```python
from build123d import *

# Parameters (mm, degrees)
SKETCH1_R           = 5
SKETCH1_R_2         = 1
SKETCH1_W           = 22
SKETCH1_H           = 12
BOSS_EXTRUDE1_DEPTH = 4


with BuildPart() as part:
    # Sketch1 → Boss-Extrude1 (new body)
    with BuildSketch(Plane.XY):
        with BuildLine():
            Line((0, 15), (200, 12.5))
            ThreePointArc((200, 12.5), (212.5, 0), (200, -12.5))
            Line((200, -12.5), (0, -15))
            ThreePointArc((0, -15), (-15, 0), (0, 15))
        make_face()
        Circle(SKETCH1_R, mode=Mode.SUBTRACT)
        with Locations((208.5, 0)):
            Circle(SKETCH1_R_2, mode=Mode.SUBTRACT)
        with Locations((181.5, 0)):
            Circle(SKETCH1_R_2, mode=Mode.SUBTRACT)
        with Locations((195, 0)):
            Rectangle(SKETCH1_W, SKETCH1_H, mode=Mode.SUBTRACT)
    extrude(amount=BOSS_EXTRUDE1_DEPTH)


solid = part.part
```
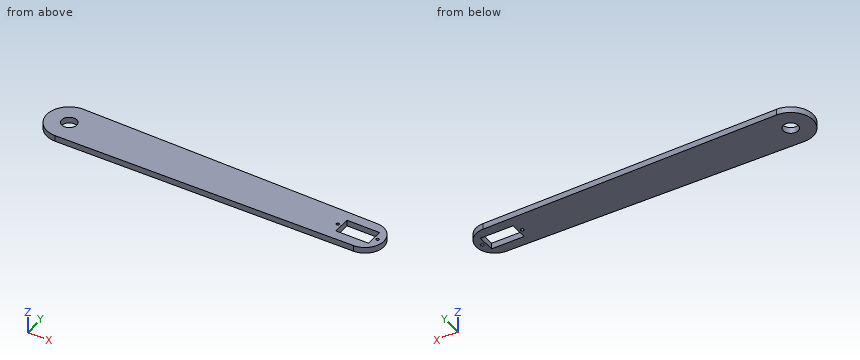
Can you work these out from the model? Positions are in its coordinate system, mm. Round coordinates to 2 decimals unless told otherwise and drop trailing zeros. Order: outer loops, then holes, each group sorted by start corner. A loop starts at its lowest first (then second) coordinate and runs counter-clockwise, first axis right, second up. Notation, with made-up numbers: (12, -34) -> (58, -34) arc R12 ccw to (58, -28) -> close; hole circle Ø1 at (-31.75, 41.25). An arc over 180 degrees is marked (long way). Return JSON: item names as keys, results as strings. Group by question number.
1. If we section it at B-B, the plane x = 124: Write out the boundary of the cut face in (y, z), then the cut area to 3 significant figures.
2. I need wall thicknesses on line 1 (Y direction, x = 0, z = 2.3); line 2 (X direction, y = 0.75, z = 1.65); line 3 (X direction, y = 3.5, z = 2.95). Which ranges of each line are inside material? Lowest first, please. Write a range as [from, to].
3. If we section it at A-A, the plane z = 3.3: Write out the boundary of the cut face in (x, y), then the cut area to 3 significant figures.
4. Will these pins go through, and if not, where does the flat tip stop? pin 1 (6 mm diameter, centred on x = 183, y = 4, fed in from -Z); pin 2 (2 mm diameter, centred on x = 197.5, z = 1.5, fed in from +Y); pin 3 (2 mm diameter, centred on y = 3, z = 1.5, fed in from -X); pin 4 (2 mm diameter, centred on y = -2.5, z = 2.5, fed in from +X).
5. If we section it at C-C, the plane y = -9.75: Write out the boundary of the cut face in (x, z), then the cut area to 3 significant figures.
Output values:
{
 "1": {"outline": "(-13.45, 0) -> (13.45, 0) -> (13.45, 4) -> (-13.45, 4) -> close", "area": "108 mm²"},
 "2": {"line 1": "[-15, -5], [5, 15]", "line 2": "[-14.98, -4.94], [4.94, 180.84], [182.16, 184], [206, 207.84], [209.16, 212.48]", "line 3": "[-14.59, -3.57], [3.57, 184], [206, 212]"},
 "3": {"outline": "(0, -15) -> (200, -12.5) arc R12.5 ccw to (200, 12.5) -> (0, 15) arc R15 ccw to start; hole circle Ø10 at (0, 0); hole circle Ø2 at (181.5, 0); hole (184, -6) -> (206, -6) -> (206, 6) -> (184, 6) -> close; hole circle Ø2 at (208.5, 0)", "area": "5,750 mm²"},
 "4": {"pin 1": "z = 0", "pin 2": "y = 12.54", "pin 3": "x = -14.87", "pin 4": "x = 212.41"},
 "5": {"outline": "(-11.4, 0) -> (207.82, 0) -> (207.82, 4) -> (-11.4, 4) -> close", "area": "877 mm²"}
}
